from build123d import *

# Parameters (mm, degrees)
F1_DEPTH = 25
F2_R     = 9.25
F3_DEPTH = 10
F4_SIZE  = 5
F6_DEPTH = 10


with BuildPart() as f1:
    # F0 (on Top) → F1 (new body)
    with BuildSketch(Plane.XY):
        with BuildLine():
            Line((17.320508, 30), (-17.320508, 30))
            ThreePointArc((-17.320508, 30), (-34.641016, 20), (-34.641016, 0))
            Line((-34.641016, 0), (-17.320508, -30))
            ThreePointArc((-17.320508, -30), (0, -40), (17.320508, -30))
            Line((17.320508, -30), (34.641016, 0))
            ThreePointArc((34.641016, 0), (34.641016, 20), (17.320508, 30))
        make_face()
    extrude(amount=F1_DEPTH)

    # F2 (on face) → F3 (cut)
    with BuildSketch(Plane.XY.offset(25)):
        with Locations((-20.78461, 12)):
            Circle(F2_R)
        with Locations((0, -24)):
            Circle(F2_R)
        with Locations((20.78461, 12)):
            Circle(F2_R)
        with Locations((0, 12)):
            Circle(F2_R)
        with Locations((-10.392305, -6)):
            Circle(F2_R)
        with Locations((10.392305, -6)):
            Circle(F2_R)
    extrude(amount=-F3_DEPTH, mode=Mode.SUBTRACT)

    # F4
    f4_edges = [f1.edges().sort_by_distance(p)[0] for p in [
        (25.980762, -15, 25),
    ]]
    chamfer(f4_edges, length=F4_SIZE)

    # F5 (on face) → F6 (cut)
    with BuildSketch(Plane(origin=(0, 0, 0), x_dir=(1, 0, 0), z_dir=(0, 0, -1))):
        with BuildLine():
            ThreePointArc((12.990381, 27.5), (0, 35), (-12.990381, 27.5))
            Line((-12.990381, 27.5), (-30.310889, -2.5))
            ThreePointArc((-30.310889, -2.5), (-30.310889, -17.5), (-17.320508, -25))
            Line((-17.320508, -25), (17.320508, -25))
            ThreePointArc((17.320508, -25), (30.310889, -17.5), (30.310889, -2.5))
            Line((30.310889, -2.5), (12.990381, 27.5))
        make_face()
    extrude(amount=-F6_DEPTH, mode=Mode.SUBTRACT)


solid = f1.part
Read the model definition and answer for the solid it produces. Units are mm, in the model's axes. A direction names the side the tool comes from. Give positions to 0.01 mm unless a question says otherwise; leave off trailing zeros. Write each loop counter-clockwise with the first axis right and the second up, starting at its lowest first coordinate (ties: lowest second). Pieces come first, ordered by that corner, then holes. Notation, with made-up numbers: (28.5, -11) -> (34.5, -11) arc R8 ccw to (34.5, -4) -> close; hole circle Ø5 at (38.5, 38). An arc over 180 degrees is marked (long way). Answer as a JSON object with one key per item and string values. Group by question number.
1) Each of these flat-tipped pins is pushed along its axis until it touches: P1, Ø15, axis at x = 0, y = -24, coming from the +Z side; P2, Ø12, axis at y = -3, z = 17, coming from the -X side; P3, Ø8, axis at x = 5, z = 4.5, coming from the -Y side (3 decimals). Where does it stop, or does it pass through?
2) Find section A-A (z = 19). Write down the section's boundary in (x, y).
3) Consider L1, parallel to Y at x = -17, z = 22; L2, parallel to Y at x = 8.5, z = 23; L3, parallel to Y at x = 18, z = 23. Determine where each line is inside the solid, lowest interval first. Write a range as from..to.
4) Find section C-C (x = 0). Write down the section's boundary in (y, z), and give its area (3 significant figures).
5) Find section B-B (z = 8.5). Write down the section's boundary in (x, y), and give its area (3 significant figures).
6) The mould has two halves that part along X. Classify faces 4 (the flat face through (23.725, -13.978, 22.465)), 5 (the flat face through (0, 30, 10)), 6 (the flat face through (21.77, -12.29, 4.93)): +X half, -X half, draft (parallel to the pull), parting line (faces both ways), or undercut.
7) A tool of negligible diameter and unlimited length cuts with its end or side. For faces 1 (the flat face through (0, -24, 15)), 2 (the flat face through (-26.1, -14.79, 9.86)), 3 (the flat face through (0, 25, 5)), from which of +Z, -Z, +X, -X, +Y, -Y can it reach the whole face along a straight path? Write none if from no direction.
8) Find section D-D (y = -24). Write down the section's boundary in (x, z).
Values follow:
{
 "1": {"P1": "stops at z = 15", "P2": "stops at x = -36.06", "P3": "stops at y = -39.975"},
 "2": {"outline": "(-34.64, 0) -> (-17.32, -30) arc R20 ccw to (17.32, -30) -> (34.64, 0) arc R20 ccw to (17.32, 30) -> (-17.32, 30) arc R20 ccw to start; hole circle Ø18.5 at (-20.78, 12); hole circle Ø18.5 at (-10.39, -6); hole circle Ø18.5 at (0, -24); hole circle Ø18.5 at (0, 12); hole circle Ø18.5 at (10.39, -6); hole circle Ø18.5 at (20.78, 12)"},
 "3": {"L1": "y = -26.56..-12.47, 0.47..3.56, 20.44..28", "L2": "y = -34.72..-27.65, -20.35..-15.05, 3.05..8.35, 15.65..27", "L3": "y = -22.82..-11.26, -0.74..3.18, 20.82..26.99"},
 "4": {"outline": "(-40, 0) -> (-35, 0) -> (-35, 10) -> (25, 10) -> (25, 0) -> (30, 0) -> (30, 20) -> (25, 25) -> (21.25, 25) -> (21.25, 15) -> (2.75, 15) -> (2.75, 25) -> (-14.75, 25) -> (-14.75, 15) -> (-33.25, 15) -> (-33.25, 25) -> (-35, 25) -> (-40, 20) -> close", "area": "755 mm2"},
 "5": {"outline": "(-34.64, 0) -> (-17.32, -30) arc R20 ccw to (17.32, -30) -> (34.64, 0) arc R20 ccw to (17.32, 30) -> (-17.32, 30) arc R20 ccw to start; hole (-30.31, 2.5) -> (-12.99, -27.5) arc R15 ccw to (12.99, -27.5) -> (30.31, 2.5) arc R15 ccw to (17.32, 25) -> (-17.32, 25) arc R15 ccw to start", "area": "1,070 mm2"},
 "6": {"face 4": "+X half", "face 5": "draft", "face 6": "undercut"},
 "7": {"face 1": "+Z", "face 2": "+Z, -Z, -X, -Y", "face 3": "-Z"},
 "8": {"outline": "(-20.78, 0) -> (-15.01, 0) -> (-15.01, 10) -> (15.01, 10) -> (15.01, 0) -> (20.78, 0) -> (20.78, 20) -> (15.01, 25) -> (9.25, 25) -> (9.25, 15) -> (-9.25, 15) -> (-9.25, 25) -> (-15.01, 25) -> (-20.78, 20) -> close"}
}
